```python
from build123d import *

# Parameters (mm, degrees)
BOSS_EXTRUDE1_DEPTH            = 35
SKETCH2_R                      = 2.6
SKETCH2_R_2                    = 1.55
BOSS_EXTRUDE3_DEPTH            = 5
CUT_EXTRUDE1_REACH             = 109.936
CUT_EXTRUDE1_DIRECTION_2_DEPTH = 108.935664458
CUT_EXTRUDE2_REACH             = 109.936
CUT_EXTRUDE2_DIRECTION_2_DEPTH = 108.935664458
FILLET1_R                      = 2
SKETCH6_R                      = 1.55
BOSS_EXTRUDE4_DEPTH            = 1


with BuildPart() as part:
    # Sketch1 → Boss-Extrude1 (new body)
    with BuildSketch(Plane(origin=(0, 0, 0), x_dir=(1, 0, 0), z_dir=(0, 1, 0))):
        Polygon((-13.5, 0), (0, 92.188031325), (13.5, 0), (14.489447114, 0.144894471), (0, 99.089605913), (-14.489447114, 0.144894471), align=None)
    extrude(amount=BOSS_EXTRUDE1_DEPTH)

    # Sketch2 → Boss-Extrude3 (add)
    # profile 1 of 10: a face of its own
    with BuildSketch(Plane(origin=(0, 0, 0), x_dir=(1, 0, 0), z_dir=(0, 1, 0))):
        with Locations((11.916884617, -0.231831154)):
            Circle(SKETCH2_R)
        with Locations(Location((11.916884617, -0.231831154, 0), (0, 0, 270))):
            Circle(SKETCH2_R_2, mode=Mode.SUBTRACT)
    # profile 2 of 10: a face of its own
    with BuildSketch(Plane(origin=(0, 0, 0), x_dir=(1, 0, 0), z_dir=(0, 1, 0))):
        with Locations((9.888362021, 13.620428448)):
            Circle(SKETCH2_R)
        with Locations(Location((9.888362021, 13.620428448, 0), (0, 0, 270))):
            Circle(SKETCH2_R_2, mode=Mode.SUBTRACT)
    # profile 3 of 10: a face of its own
    with BuildSketch(Plane(origin=(0, 0, 0), x_dir=(1, 0, 0), z_dir=(0, 1, 0))):
        with Locations((7.859839425, 27.47268805)):
            Circle(SKETCH2_R)
        with Locations(Location((7.859839425, 27.47268805, 0), (0, 0, 270))):
            Circle(SKETCH2_R_2, mode=Mode.SUBTRACT)
    # profile 4 of 10: a face of its own
    with BuildSketch(Plane(origin=(0, 0, 0), x_dir=(1, 0, 0), z_dir=(0, 1, 0))):
        with Locations((5.831316829, 41.324947652)):
            Circle(SKETCH2_R)
        with Locations(Location((5.831316829, 41.324947652, 0), (0, 0, 270))):
            Circle(SKETCH2_R_2, mode=Mode.SUBTRACT)
    # profile 5 of 10: a face of its own
    with BuildSketch(Plane(origin=(0, 0, 0), x_dir=(1, 0, 0), z_dir=(0, 1, 0))):
        with Locations((3.802794233, 55.177207254)):
            Circle(SKETCH2_R)
        with Locations(Location((3.802794233, 55.177207254, 0), (0, 0, 270))):
            Circle(SKETCH2_R_2, mode=Mode.SUBTRACT)
    # profile 6 of 10: a face of its own
    with BuildSketch(Plane(origin=(0, 0, 0), x_dir=(1, 0, 0), z_dir=(0, 1, 0))):
        with Locations((-11.916884617, -0.231831154)):
            Circle(SKETCH2_R)
        with Locations(Location((-11.916884617, -0.231831154, 0), (0, 0, 90))):
            Circle(SKETCH2_R_2, mode=Mode.SUBTRACT)
    # profile 7 of 10: a face of its own
    with BuildSketch(Plane(origin=(0, 0, 0), x_dir=(1, 0, 0), z_dir=(0, 1, 0))):
        with Locations((-9.888362021, 13.620428448)):
            Circle(SKETCH2_R)
        with Locations(Location((-9.888362021, 13.620428448, 0), (0, 0, 90))):
            Circle(SKETCH2_R_2, mode=Mode.SUBTRACT)
    # profile 8 of 10: a face of its own
    with BuildSketch(Plane(origin=(0, 0, 0), x_dir=(1, 0, 0), z_dir=(0, 1, 0))):
        with Locations((-7.859839425, 27.47268805)):
            Circle(SKETCH2_R)
        with Locations(Location((-7.859839425, 27.47268805, 0), (0, 0, 90))):
            Circle(SKETCH2_R_2, mode=Mode.SUBTRACT)
    # profile 9 of 10: a face of its own
    with BuildSketch(Plane(origin=(0, 0, 0), x_dir=(1, 0, 0), z_dir=(0, 1, 0))):
        with Locations((-5.831316829, 41.324947652)):
            Circle(SKETCH2_R)
        with Locations(Location((-5.831316829, 41.324947652, 0), (0, 0, 90))):
            Circle(SKETCH2_R_2, mode=Mode.SUBTRACT)
    # profile 10 of 10: a face of its own
    with BuildSketch(Plane(origin=(0, 0, 0), x_dir=(1, 0, 0), z_dir=(0, 1, 0))):
        with Locations((-3.802794233, 55.177207254)):
            Circle(SKETCH2_R)
        with Locations(Location((-3.802794233, 55.177207254, 0), (0, 0, 90))):
            Circle(SKETCH2_R_2, mode=Mode.SUBTRACT)
    boss_extrude3 = extrude(amount=BOSS_EXTRUDE3_DEPTH)

    # Cut-Extrude1: up to this face of the body (flat: up to its plane)
    cut_extrude1_end = Plane(part.part.faces().sort_by_distance((-6.685224914, 17.936553529, -46.536348085))[0])
    # Sketch4 → Cut-Extrude1 (cut, up to the picked face)
    with BuildSketch(Plane(origin=(0.283424505, 0, 1.935433121), x_dir=(0.9894471144188783, 0, -0.14489447114419254), z_dir=(0.14489447114419252, 0, 0.9894471144188782)), mode=Mode.PRIVATE) as cut_extrude1_sk1:
        Polygon((13.357536045, 5), (9.157536045, 5), (9.157536045, 1.475781549), align=None)
    cut_extrude1_tool1 = split(extrude(cut_extrude1_sk1.sketch, amount=-CUT_EXTRUDE1_REACH, mode=Mode.PRIVATE), bisect_by=cut_extrude1_end, keep=Keep.BOTH, mode=Mode.PRIVATE)
    cut_extrude1 = cut_extrude1_tool1.solids().sort_by(Axis((10.729548, 3.825261, 0.405705), (-0.14489447114419252, 0, -0.9894471144188782)))[0]
    add(cut_extrude1, mode=Mode.SUBTRACT)

    # Sketch4 → Cut-Extrude1 direction 2 (cut)
    with BuildSketch(Plane(origin=(0.283424505, 0, 1.935433121), x_dir=(0.9894471144188783, 0, -0.14489447114419254), z_dir=(0.14489447114419252, 0, 0.9894471144188782))):
        Polygon((13.357536045, 5), (9.157536045, 5), (9.157536045, 1.475781549), align=None)
    cut_extrude1_direction_2 = extrude(amount=CUT_EXTRUDE1_DIRECTION_2_DEPTH, mode=Mode.SUBTRACT)

    # Cut-Extrude2: up to this face of the body (flat: up to its plane)
    cut_extrude2_end = Plane(part.part.faces().sort_by_distance((6.685224914, 17.936553529, -46.536348085))[0])
    # Sketch5 → Cut-Extrude2 (cut, up to the picked face)
    with BuildSketch(Plane(origin=(-0.283424505, 0, 1.935433121), x_dir=(0.9894471144188784, 0, 0.14489447114419146), z_dir=(-0.14489447114419146, 0, 0.9894471144188784)), mode=Mode.PRIVATE) as cut_extrude2_sk1:
        Polygon((-9.157536045, 5), (-9.157536045, 1.475781549), (-13.357536045, 5), align=None)
    cut_extrude2_tool1 = split(extrude(cut_extrude2_sk1.sketch, amount=-CUT_EXTRUDE2_REACH, mode=Mode.PRIVATE), bisect_by=cut_extrude2_end, keep=Keep.BOTH, mode=Mode.PRIVATE)
    cut_extrude2 = cut_extrude2_tool1.solids().sort_by(Axis((-10.729548, 3.825261, 0.405705), (0.14489447114419146, 0, -0.9894471144188784)))[0]
    add(cut_extrude2, mode=Mode.SUBTRACT)

    # Sketch5 → Cut-Extrude2 direction 2 (cut)
    with BuildSketch(Plane(origin=(-0.283424505, 0, 1.935433121), x_dir=(0.9894471144188784, 0, 0.14489447114419146), z_dir=(-0.14489447114419146, 0, 0.9894471144188784))):
        Polygon((-9.157536045, 5), (-9.157536045, 1.475781549), (-13.357536045, 5), align=None)
    cut_extrude2_direction_2 = extrude(amount=CUT_EXTRUDE2_DIRECTION_2_DEPTH, mode=Mode.SUBTRACT)

    # Mirror2: Boss-Extrude3, Cut-Extrude1, Cut-Extrude1 direction 2, Cut-Extrude2, Cut-Extrude2 direction 2 across plane
    add(boss_extrude3.mirror(Plane.ZX.offset(17.5)))
    add(cut_extrude1.mirror(Plane.ZX.offset(17.5)), mode=Mode.SUBTRACT)
    add(cut_extrude1_direction_2.mirror(Plane.ZX.offset(17.5)), mode=Mode.SUBTRACT)
    add(cut_extrude2.mirror(Plane.ZX.offset(17.5)), mode=Mode.SUBTRACT)
    add(cut_extrude2_direction_2.mirror(Plane.ZX.offset(17.5)), mode=Mode.SUBTRACT)

    # Fillet1
    # the kernel refuses this fillet: 2 mm, written as the material it adds along each edge
    with BuildSketch(Plane(origin=(13.5, 5, 0), x_dir=(0, 1, 0), z_dir=(0.9894471144188783, 0, -0.1448944711441925))) as fillet1_piece_1_section:
        with BuildLine():
            CenterArc((FILLET1_R, FILLET1_R), FILLET1_R, 180, 90)
            Line((0, FILLET1_R), (0, 0))
            Line((0, 0), (FILLET1_R, 0))
        make_face()
    fillet1_piece_1 = extrude(amount=6, mode=Mode.PRIVATE)
    fillet1_piece_1 = fillet1_piece_1 & Plane(origin=(11.916884617, 5.699977741, 0.231831154), x_dir=(1, 0, 0), z_dir=(0, -1, 0)) * Cylinder(2.6, 20, mode=Mode.PRIVATE)
    add(fillet1_piece_1)
    with BuildSketch(Plane(origin=(13.5, 30, 0), x_dir=(0, -1, 0), z_dir=(0.9894471144188783, 0, -0.1448944711441925))) as fillet1_piece_2_section:
        with BuildLine():
            CenterArc((FILLET1_R, -FILLET1_R), FILLET1_R, 90, 90)
            Line((0, -FILLET1_R), (0, 0))
            Line((0, 0), (FILLET1_R, 0))
        make_face()
    fillet1_piece_2 = extrude(amount=6, mode=Mode.PRIVATE)
    fillet1_piece_2 = fillet1_piece_2 & Plane(origin=(11.916884617, 29.30002226, 0.231831154), x_dir=(1, 0, 0), z_dir=(0, 1, 0)) * Cylinder(2.6, 20, mode=Mode.PRIVATE)
    add(fillet1_piece_2)
    with BuildSketch(Plane(origin=(-19.436682687, 30, -0.869366827), x_dir=(0, -1, 0), z_dir=(0.9894471144188784, 0, 0.1448944711441914))) as fillet1_piece_3_section:
        with BuildLine():
            CenterArc((FILLET1_R, -FILLET1_R), FILLET1_R, 90, 90)
            Line((0, -FILLET1_R), (0, 0))
            Line((0, 0), (FILLET1_R, 0))
        make_face()
    fillet1_piece_3 = extrude(amount=6, mode=Mode.PRIVATE)
    fillet1_piece_3 = fillet1_piece_3 & Plane(origin=(-11.916884617, 29.777637105, 0.231831154), x_dir=(1, 0, 0), z_dir=(0, 1, 0)) * Cylinder(2.6, 21, mode=Mode.PRIVATE)
    add(fillet1_piece_3)
    with BuildSketch(Plane(origin=(-19.436682687, 5, -0.869366827), x_dir=(-0.1448944711441914, 0, 0.9894471144188784), z_dir=(0.9894471144188784, 0, 0.1448944711441914))) as fillet1_piece_4_section:
        with BuildLine():
            CenterArc((FILLET1_R, -FILLET1_R), FILLET1_R, 90, 90)
            Line((0, -FILLET1_R), (0, 0))
            Line((0, 0), (FILLET1_R, 0))
        make_face()
    fillet1_piece_4 = extrude(amount=6, mode=Mode.PRIVATE)
    fillet1_piece_4 = fillet1_piece_4 & Plane(origin=(-11.916884617, 5.222362792, 0.231831154), x_dir=(1, 0, 0), z_dir=(0, -1, 0)) * Cylinder(2.6, 21, mode=Mode.PRIVATE)
    add(fillet1_piece_4)

    # Sketch6 → Boss-Extrude4 (add)
    with BuildSketch(Plane.XZ):
        with Locations(Location((3.802794233, -55.177207254, 0), (0, 0, 270))):
            Circle(SKETCH6_R)
        with Locations(Location((-3.802794233, -55.177207254, 0), (0, 0, 270))):
            Circle(SKETCH6_R)
        with Locations(Location((-5.831316829, -41.324947652, 0), (0, 0, 270))):
            Circle(SKETCH6_R)
        with Locations(Location((5.831316829, -41.324947652, 0), (0, 0, 270))):
            Circle(SKETCH6_R)
        with Locations(Location((7.859839425, -27.47268805, 0), (0, 0, 270))):
            Circle(SKETCH6_R)
        with Locations(Location((-7.859839425, -27.47268805, 0), (0, 0, 270))):
            Circle(SKETCH6_R)
        with Locations(Location((-9.888362021, -13.620428448, 0), (0, 0, 270))):
            Circle(SKETCH6_R)
        with Locations(Location((9.888362021, -13.620428448, 0), (0, 0, 270))):
            Circle(SKETCH6_R)
        with Locations(Location((11.916884617, 0.231831154, 0), (0, 0, 270))):
            Circle(SKETCH6_R)
        with Locations(Location((-11.916884617, 0.231831154, 0), (0, 0, 270))):
            Circle(SKETCH6_R)
    extrude(amount=-BOSS_EXTRUDE4_DEPTH)


solid = part.part
```
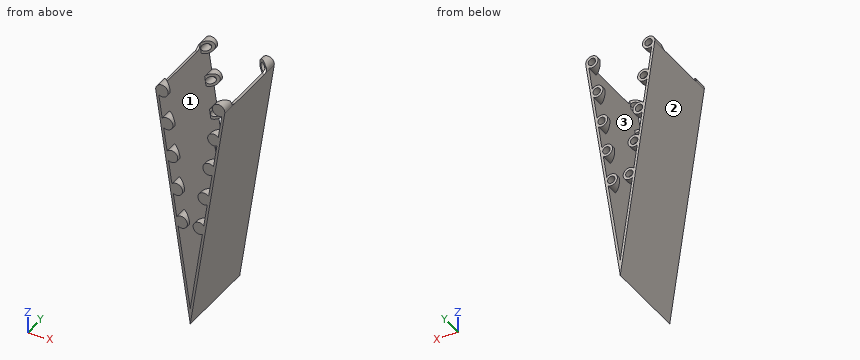
Verification items for the finished model (mm, model axes). Face numbers are marked on the shaded views. Give positions to 0.01 mm unless a question says otherwise; leave off trailing zeros. Order: outer loops, then holes, each group sorted by start corner. A loop starts at its lowest first (then second) coordinate and runs counter-clockwise, first axis right, second up. Notation, with made-up numbers: (9, 76.25) -> (49, 76.25) arc R22 cw to (49, 96.25) -> close; hole circle Ø4 at (-37, 42.25). An arc over 180 degrees is marked (long way). One line per item, written item: value.
(1) Sectioned sample at B-B on z = -65. Record the cut outline in (x, y).
Final values:
outline: (-4.99, 0) -> (-3.98, 0) -> (-3.98, 35) -> (-4.99, 35) -> close; (3.98, 0) -> (4.99, 0) -> (4.99, 35) -> (3.98, 35) -> close
(2) Draft check along Z on the marked faces 1, 2 and 3. Enter one of: pulls with the +Z half, pulls with the -Z half, needs draft (parallel to the pull), parting line crosses it, or undercut.
Final values:
face 1: undercut
face 2: pulls with the -Z half
face 3: undercut
(3) Sectioned sample at A-A on y = 19. Record the cut outline in (x, z).
Final values:
outline: (-14.49, -0.14) -> (0, -99.09) -> (14.49, -0.14) -> (13.5, 0) -> (0, -92.19) -> (-13.5, 0) -> close
(4) Scan lines: line 1 along X through (y, z) = (24.5, -45.5); line 2 along X through (y, z) = (6, -41). Record each from-to range of solid material in increasing order. Write a range as [from, to].
Final values:
line 1: [-7.85, -6.84], [6.84, 7.85]
line 2: [-8.51, -7.5], [7.5, 8.51]
(5) Gauge pin test, flat ends, axial feed: pin 1 (0.9 mm diameter, centred on x = 4.5, z = -55.5, fed in from +Y); pin 2 (3.5 mm diameter, centred on x = -11.92, z = 0.23, fed in from +Y); pin 3 (10 mm diameter, centred on y = 20, z = -81, fed in from -X); pin 4 (8 mm diameter, centred on y = 29.5, z = -58, fed in from -X). Record the tip position at first contact, or that the pin passes through.
Final values:
pin 1: y = 1
pin 2: y = 35
pin 3: x = -3.38
pin 4: x = -6.6
